Source: CAD feature listing. Evaluate the final solid. Frame: model axes, mm. Round coordinates to 2 decimals unless told otherwise and drop trailing zeros. Write each loop counter-clockwise with the first axis right and the second up, starting at its lowest first coordinate (ties: lowest second). Pieces come first, ordered by that corner, then holes. Notation, with made-up numbers: M 48,84.25 L 100,84.25 A19 cw 100,88.25 Z; hole C -26.75,66.25 d9. An arc over 180 degrees is marked long. Use a Markdown table: item, result.
```python
from build123d import *

# Parameters (mm, degrees)
F1_DEPTH = 4
F2_D     = 3


with BuildPart() as f1:
    # F0 (on Top) → F1 (new body)
    with BuildSketch(Plane.XY):
        with BuildLine():
            ThreePointArc((-52.18448, 159.947554), (-35.666397, 135.226495), (-29.866017, 106.066017))
            ThreePointArc((-29.866017, 106.066017), (-76.90554, 35.666397), (-159.947554, 52.18448))
            Line((-159.947554, 52.18448), (-167.018622, 45.113413))
            ThreePointArc((-167.018622, 45.113413), (-73.078705, 26.427601), (-19.866017, 106.066017))
            ThreePointArc((-19.866017, 106.066017), (-26.427601, 139.053329), (-45.113413, 167.018622))
            Line((-45.113413, 167.018622), (-52.18448, 159.947554))
        make_face()
        with BuildLine():
            ThreePointArc((-159.947554, 52.18448), (-159.947554, 159.947554), (-52.18448, 159.947554))
            Line((-52.18448, 159.947554), (-45.113413, 167.018622))
            ThreePointArc((-45.113413, 167.018622), (-167.018622, 167.018622), (-167.018622, 45.113413))
            Line((-167.018622, 45.113413), (-159.947554, 52.18448))
        make_face()
        with BuildLine():
            ThreePointArc((45.113413, 167.018622), (0, 148.813707), (-45.113413, 167.018622))
            ThreePointArc((-45.113413, 167.018622), (-26.427601, 139.053329), (-19.866017, 106.066017))
            ThreePointArc((-19.866017, 106.066017), (-73.078705, 26.427601), (-167.018622, 45.113413))
            ThreePointArc((-167.018622, 45.113413), (-148.813707, 0), (-167.018622, -45.113413))
            ThreePointArc((-167.018622, -45.113413), (-73.078705, -26.427601), (-19.866017, -106.066017))
            ThreePointArc((-19.866017, -106.066017), (-26.427601, -139.053329), (-45.113413, -167.018622))
            ThreePointArc((-45.113413, -167.018622), (0, -148.813707), (45.113413, -167.018622))
            ThreePointArc((45.113413, -167.018622), (45.113413, -45.113413), (167.018622, -45.113413))
            ThreePointArc((167.018622, -45.113413), (148.813707, 0), (167.018622, 45.113413))
            ThreePointArc((167.018622, 45.113413), (45.113413, 45.113413), (45.113413, 167.018622))
        make_face()
        with BuildLine():
            Line((52.18448, 159.947554), (45.113413, 167.018622))
            ThreePointArc((45.113413, 167.018622), (45.113413, 45.113413), (167.018622, 45.113413))
            Line((167.018622, 45.113413), (159.947554, 52.18448))
            ThreePointArc((159.947554, 52.18448), (52.18448, 52.18448), (52.18448, 159.947554))
        make_face()
        with BuildLine():
            ThreePointArc((192.266017, 106.066017), (139.053329, 185.704433), (45.113413, 167.018622))
            Line((45.113413, 167.018622), (52.18448, 159.947554))
            ThreePointArc((52.18448, 159.947554), (135.226495, 176.465638), (182.266017, 106.066017))
            ThreePointArc((182.266017, 106.066017), (176.465638, 76.90554), (159.947554, 52.18448))
            Line((159.947554, 52.18448), (167.018622, 45.113413))
            ThreePointArc((167.018622, 45.113413), (185.704433, 73.078705), (192.266017, 106.066017))
        make_face()
        with BuildLine():
            Line((159.947554, -52.18448), (167.018622, -45.113413))
            ThreePointArc((167.018622, -45.113413), (45.113413, -45.113413), (45.113413, -167.018622))
            Line((45.113413, -167.018622), (52.18448, -159.947554))
            ThreePointArc((52.18448, -159.947554), (52.18448, -52.18448), (159.947554, -52.18448))
        make_face()
        with BuildLine():
            ThreePointArc((192.266017, -106.066017), (185.704433, -73.078705), (167.018622, -45.113413))
            Line((167.018622, -45.113413), (159.947554, -52.18448))
            ThreePointArc((159.947554, -52.18448), (176.465638, -76.90554), (182.266017, -106.066017))
            ThreePointArc((182.266017, -106.066017), (135.226495, -176.465638), (52.18448, -159.947554))
            Line((52.18448, -159.947554), (45.113413, -167.018622))
            ThreePointArc((45.113413, -167.018622), (139.053329, -185.704433), (192.266017, -106.066017))
        make_face()
        with BuildLine():
            Line((-159.947554, -52.18448), (-167.018622, -45.113413))
            ThreePointArc((-167.018622, -45.113413), (-167.018622, -167.018622), (-45.113413, -167.018622))
            Line((-45.113413, -167.018622), (-52.18448, -159.947554))
            ThreePointArc((-52.18448, -159.947554), (-159.947554, -159.947554), (-159.947554, -52.18448))
        make_face()
        with BuildLine():
            ThreePointArc((-19.866017, -106.066017), (-73.078705, -26.427601), (-167.018622, -45.113413))
            Line((-167.018622, -45.113413), (-159.947554, -52.18448))
            ThreePointArc((-159.947554, -52.18448), (-76.90554, -35.666397), (-29.866017, -106.066017))
            ThreePointArc((-29.866017, -106.066017), (-35.666397, -135.226495), (-52.18448, -159.947554))
            Line((-52.18448, -159.947554), (-45.113413, -167.018622))
            ThreePointArc((-45.113413, -167.018622), (-26.427601, -139.053329), (-19.866017, -106.066017))
        make_face()
    extrude(amount=F1_DEPTH)

    # F2 (through all)
    with Locations(Plane(origin=(0, 0, 0), x_dir=(1, 0, 0), z_dir=(0, 0, -1))):
        with Locations((-163.483088, 163.483088), (-48.648947, 163.483088), (-48.648947, 48.648947), (-163.483088, 48.648947), (-163.483088, -48.648947), (-48.648947, -48.648947), (-48.648947, -163.483088), (-163.483088, -163.483088), (48.648947, -163.483088), (48.648947, -48.648947), (163.483088, -48.648947), (163.483088, -163.483088), (163.483088, 163.483088), (163.483088, 48.648947), (48.648947, 48.648947), (48.648947, 163.483088)):
            Hole(F2_D / 2)


solid = f1.part
```
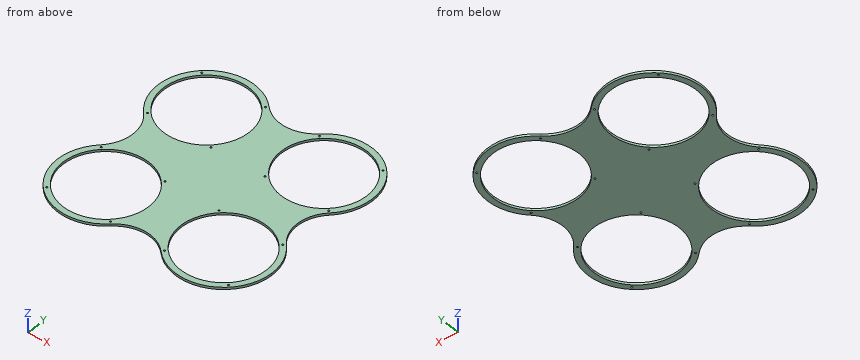
Q1. Section D-D on y = 3. Return loops of the section in (x, z).
Results are:
| item | result |
|---|---|
| outline | M -148.88,0 L 148.88,0 L 148.88,4 L -148.88,4 Z |
Q2. Line query: L1, parallel to Y at x = -57, z = 3.2; L2, parallel to Y at x = -83, z = 3.55; L3, parallel to X at y = 68, z = 3.85. Output: solid intervals per line, ascending.
Results are:
| item | result |
|---|---|
| L1 | -176.94 to -164.37, -47.77 to 47.77, 164.37 to 176.94 |
| L2 | -189.12 to -178.69, -33.44 to 33.44, 178.69 to 189.12 |
| L3 | -183.41 to -172.08, -40.06 to 40.06, 172.08 to 183.41 |
Q3. Section B-B on y = 60.5. Return loops of the section in (x, z), plus the area to 3 significant figures.
Results are:
| item | result |
|---|---|
| outline | M -179.24,0 L -167.14,0 L -167.14,4 L -179.24,4 Z; M -44.99,0 L 44.99,0 L 44.99,4 L -44.99,4 Z; M 167.14,0 L 179.24,0 L 179.24,4 L 167.14,4 Z |
| area | 457 mm^2 |
Q4. Section C-C on z = 1.35. Give the number of separate pieces and of enclosed holes in the cut face, plus the area to 3 significant figures.
Results are:
| item | result |
|---|---|
| separate pieces | 1 |
| enclosed holes | 20 |
| area | 50,900 mm^2 |
Q5. First-contact query: pin 1 Ø1.5 at (x, z) = (-6.5, 2) entering from -Y; pin 2 Ø3.5 at (x, y) = (48.65, 48.65) entering from +Z; pin 3 Ø1.5 at (y, z) = (52.5, 3) entering from -X. Flat tips, straight axial feed; report the tip coordinate or a pass-through.
Results are:
| item | result |
|---|---|
| pin 1 | y = -149.22 |
| pin 2 | z = 4 |
| pin 3 | x = -174.19 |
Q6. Section A-A on x = -109.5. Return loops of the section in (y, z), plus the area to 3 significant figures.
Results are:
| item | result |
|---|---|
| outline | M -192.2,0 L -182.19,0 L -182.19,4 L -192.2,4 Z; M -29.94,0 L 29.94,0 L 29.94,4 L -29.94,4 Z; M 182.19,0 L 192.2,0 L 192.2,4 L 182.19,4 Z |
| area | 320 mm^2 |
